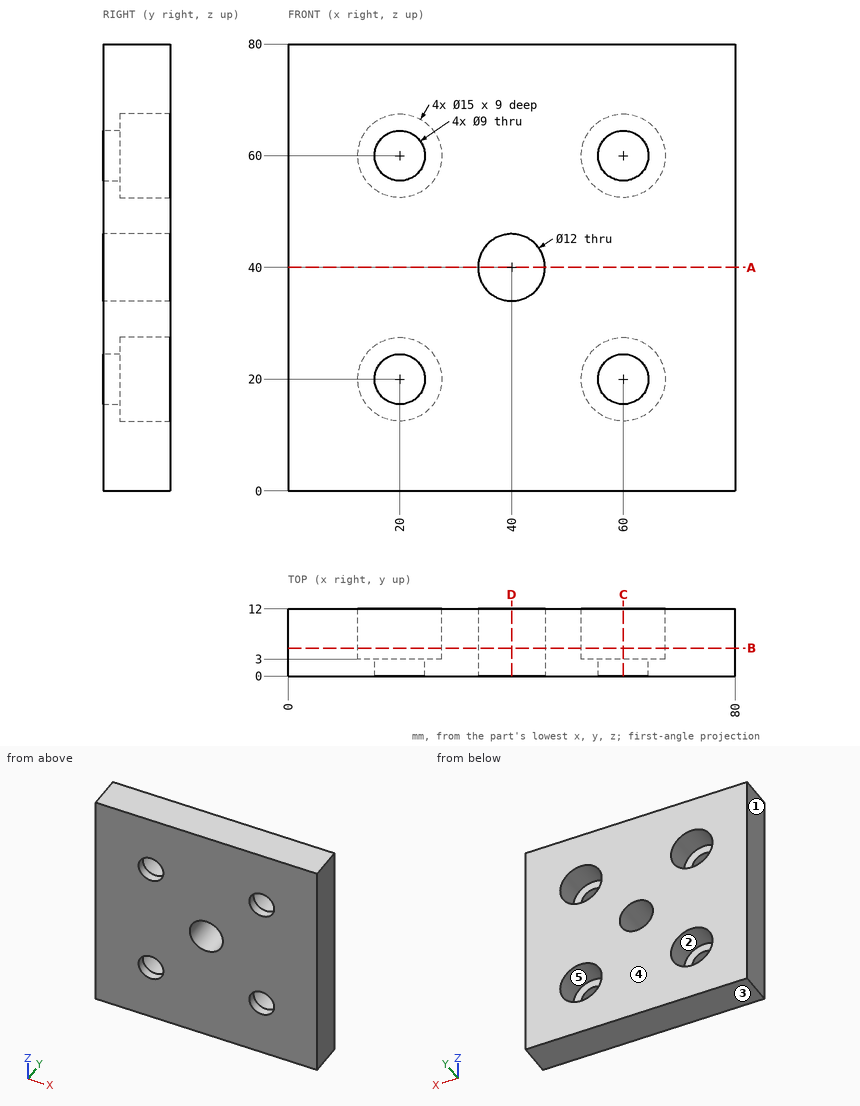
Source: three-view drawing plus pictorial views. Frame: mm from the lowest corner of the part. A direction names the side the tool comes from. Round coordinates to 2 decimals unless told otherwise and drop trailing zeros. Write each loop counter-clockwise with the first axis right and the second up, starting at its lowest first coordinate (ties: lowest second). Pieces come first, ordered by that corner, then holes. Notation, with made-up numbers: M 79,-14.75 L 113,-14.75 A22 ccw 113,13.25 Z; hole C 74.5,40.25 d10. An arc over 180 degrees is marked long. Use CSV: the item, a comma, the result in double quotes. Start each with the question number.
Q1. Pull-direction query (X, two-part tool) for the marked faces 1, 2 and 3; classes: +X half, -X half, draft (parallel to the pull), parting line (faces both ways), or undercut.
Q2. Cut plane D-D on x = 40. Output: boundary loops of the cut face in (y, z), plus the area to 3 significant figures.
Q3. Line query: line 1 (X direction, y = 1, z = 20); line 2 (X direction, y = 5.25, z = 60); line 3 (X direction, y = 3.75, z = 40). Output: solid intervals per line, ascending. Write a range as from..to.
Q4. Cut plane C-C on x = 60. Output: boundary loops of the cut face in (y, z).
Q5. Access query for the marked faces 4 and 5. Directions: +Z, -Z, +X, -X, +Y, -Y. A direction counts if a zero-diameter tool reaches every point of the face in a straight line with its end or side. Return the directions, or none.
Q6. First-contact query: P1, Ø12, axis at x = 18, z = 23, coming from the +Y side; P2, Ø7.5, axis at x = 57.5, z = 59.5, coming from the +Y side. Flat tips, straight axial feed; report the tip coordinate or a pass-through.
Q7. Cut plane B-B on y = 5. Output: boundary loops of the cut face in (x, z), plus the area to 3 significant figures.
Q8. Cut plane A-A on z = 40. Output: boundary loops of the cut face in (x, y), plus the area to 3 significant figures.
Results found:
1,face 1,"-X half"
1,face 2,"undercut"
1,face 3,"draft"
2,outline,"M 0,0 L 12,0 L 12,34 L 0,34 Z; M 0,46 L 12,46 L 12,80 L 0,80 Z"
2,area,"816 mm^2"
3,line 1,"0..15.5, 24.5..55.5, 64.5..80"
3,line 2,"0..12.5, 27.5..52.5, 67.5..80"
3,line 3,"0..34, 46..80"
4,outline,"M 0,0 L 12,0 L 12,12.5 L 3,12.5 L 3,15.5 L 0,15.5 Z; M 0,24.5 L 3,24.5 L 3,27.5 L 12,27.5 L 12,52.5 L 3,52.5 L 3,55.5 L 0,55.5 Z; M 0,64.5 L 3,64.5 L 3,67.5 L 12,67.5 L 12,80 L 0,80 Z"
5,face 4,"+Z, -Z, +X, -X, +Y"
5,face 5,"+Y"
6,P1,"y = 12"
6,P2,"y = 3"
7,outline,"M 0,0 L 80,0 L 80,80 L 0,80 Z; hole C 20,20 d15; hole C 20,60 d15; hole C 40,40 d12; hole C 60,20 d15; hole C 60,60 d15"
7,area,"5,580 mm^2"
8,outline,"M 0,0 L 34,0 L 34,12 L 0,12 Z; M 46,0 L 80,0 L 80,12 L 46,12 Z"
8,area,"816 mm^2"
